```python
from build123d import *

# Parameters (mm, degrees)
F0_W     = 147.184163332
F0_H     = 89.8508056998
F0_R     = 15.1184260195
F0_R_2   = 15.0482996588
F1_DEPTH = 76.2
F3_DEPTH = 101.6
F4_DEPTH = 12.7
F6_DEPTH = 114.301


with BuildPart() as f1:
    # F0 (on Top) → F1 (new body)
    with BuildSketch(Plane.XY):
        Rectangle(F0_W, F0_H)
        with Locations((-55.6219257414, 0)):
            Circle(F0_R, mode=Mode.SUBTRACT)
        with Locations((55.6219220161, 0)):
            Circle(F0_R_2, mode=Mode.SUBTRACT)
    extrude(amount=F1_DEPTH)

    # F2 (on face) → F3 (join)
    with BuildSketch(Plane.XZ.offset(44.9254028499)):
        with BuildLine():
            ThreePointArc((-35.903516253, 76.2), (0, 40.296483747), (35.903516253, 76.2))
            Line((35.903516253, 76.2), (-35.903516253, 76.2))
        make_face()
    extrude(amount=-F3_DEPTH)

    # F2 (on face) → F4 (join)
    with BuildSketch(Plane.XZ.offset(44.9254028499)):
        with BuildLine():
            ThreePointArc((-35.903516253, 76.2), (0, 40.296483747), (35.903516253, 76.2))
            Line((35.903516253, 76.2), (-35.903516253, 76.2))
        make_face()
    extrude(amount=F4_DEPTH)

    # F5 (on face) → F6 (cut, through all)
    with BuildSketch(Plane.XZ.offset(57.6254028499)):
        with BuildLine():
            Line((-21.3098982127, 76.2), (21.3098982127, 76.2))
            ThreePointArc((21.3098982127, 76.2), (0, 97.5098982127), (-21.3098982127, 76.2))
        make_face()
        with BuildLine():
            ThreePointArc((-21.3098982127, 76.2), (0, 54.8901017873), (21.3098982127, 76.2))
            Line((21.3098982127, 76.2), (-21.3098982127, 76.2))
        make_face()
    extrude(amount=-F6_DEPTH, mode=Mode.SUBTRACT)


solid = f1.part
```
Verification items for the finished model (mm, model axes). A direction names the side the tool comes from. Give positions to 0.01 mm unless a question says otherwise; leave off trailing zeros. Loops run counter-clockwise (first coordinate to the right, second up) from the corner with the lowest first, then second, coordinate; pieces in that order, holes last. Notation, with made-up numbers: M -11.5,-20 L 6.5,-20 A26 ccw 6.5,6 Z; hole C -36,21 d3. An arc over 180 degrees is marked long. One line per question, with ' | ' between items.
Item 1: Tool access check on faces 4 (the face through (35, 0, 76.2)), 5 (the face through (-0.789, 50.718, 40.305)). Record the directions out of +Z, -Z, +X, -X, +Y, -Y that give a thin tool (end or side, any length) a straight path to the whole face; none if there is none.
Completed:
face 4: +Z, +X, -X, +Y, -Y | face 5: -Z, +Y
Item 2: Thickness scan on line 1 (Y direction, x = 52, z = 53.5); line 2 (X direction, y = 12.5, z = 44); line 3 (Y direction, x = -62, z = 61). Record the ranges inside material, lowest first. Write a range as [from, to].
Completed:
line 1: y = [-44.93, -14.61], [14.61, 44.93] | line 2: x = [-73.59, -64.13], [-47.12, 47.24], [64, 73.59] | line 3: y = [-44.93, -13.71], [13.71, 44.93]
Item 3: Section check D-D, the plane z = 14. Record the cut outline in (x, y).
Completed:
outline: M -73.59,-44.93 L 73.59,-44.93 L 73.59,44.93 L -73.59,44.93 Z; hole C -55.62,0 d30.24; hole C 55.62,0 d30.1
Item 4: Section check A-A, the plane y = 0. Record the cut outline in (x, z), plus the area to 3 significant figures.
Completed:
outline: M -73.59,0 L -70.74,0 L -70.74,76.2 L -73.59,76.2 Z; M -40.5,0 L 40.57,0 L 40.57,76.2 L 21.31,76.2 A21.31 cw -21.31,76.2 L -40.5,76.2 Z; M 70.67,0 L 73.59,0 L 73.59,76.2 L 70.67,76.2 Z | area: 5,900 mm^2
Item 5: Section check C-C, the plane x = 0. Record the cut outline in (y, z).
Completed:
outline: M -57.63,40.3 L -44.93,40.3 L -44.93,0 L 44.93,0 L 44.93,40.3 L 56.67,40.3 L 56.67,54.89 L -57.63,54.89 Z
Item 6: Section check B-B, the plane z = 63. Record the cut outline in (x, y), plus the area to 3 significant figures.
Completed:
outline: M -73.59,-44.93 L -33.39,-44.93 L -33.39,-57.63 L -16.73,-57.63 L -16.73,56.67 L -33.39,56.67 L -33.39,44.93 L -73.59,44.93 Z; M 16.73,-57.63 L 33.39,-57.63 L 33.39,-44.93 L 73.59,-44.93 L 73.59,44.93 L 33.39,44.93 L 33.39,56.67 L 16.73,56.67 Z; hole C -55.62,0 d30.24; hole C 55.62,0 d30.1 | area: 9,600 mm^2
Item 7: Depth check by flat-ended pin: P1, Ø10, axis at x = -28.5, y = -15, coming from the -Z side; P2, Ø5, axis at x = -49.5, z = 41.5, coming from the -Y side; P3, Ø12, axis at x = -53.5, z = 56.5, coming from the +Y side. Enter the tip coordinate at first touch or a pass-through.
Completed:
P1: stops at z = 0 | P2: stops at y = -44.93 | P3: stops at y = 44.93
Item 8: Draft check along Y on faces 1 (the face through (-1, -44.925, 30)), 2 (the face through (-67.62, -9.2, 37.57)), 3 (the face through (-0.789, -51.187, 40.305)). Enter one of: +Y half, -Y half, draft (parallel to the pull), parting line (faces both ways), or undercut.
Completed:
face 1: -Y half | face 2: undercut | face 3: draft
